from build123d import *

# Parameters (mm, degrees)
SKETCH1_R           = 7
BOSS_EXTRUDE1_DEPTH = 1
SKETCH2_R           = 6.475
BOSS_EXTRUDE2_DEPTH = 2
SKETCH3_R           = 4.75
CUT_EXTRUDE1_DEPTH  = 11.344080433
CHAMFER1_SIZE       = 0.5


with BuildPart() as part:
    # Sketch1 → Boss-Extrude1 (new body)
    with BuildSketch(Plane(origin=(0, 0, 0), x_dir=(1, 0, 0), z_dir=(0, 1, 0))):
        with Locations(Location((0, 0, 0), (0, 0, 270))):
            Circle(SKETCH1_R)
    extrude(amount=BOSS_EXTRUDE1_DEPTH)

    # Sketch2 → Boss-Extrude2 (add)
    with BuildSketch(Plane(origin=(0, 1, 0), x_dir=(1, 0, 0), z_dir=(0, 1, 0))):
        with Locations(Location((0, 0, 0), (0, 0, 270))):
            Circle(SKETCH2_R)
    extrude(amount=BOSS_EXTRUDE2_DEPTH)

    # Sketch3 → Cut-Extrude1 (cut, through all)
    with BuildSketch(Plane.XZ):
        with Locations(Location((0, 0, 0), (0, 0, 270))):
            Circle(SKETCH3_R)
    extrude(amount=-CUT_EXTRUDE1_DEPTH, mode=Mode.SUBTRACT)

    # Chamfer1
    chamfer1_edges = [part.edges().sort_by_distance(p)[0] for p in [
        (0, 0, 4.75),
    ]]
    chamfer(chamfer1_edges, length=CHAMFER1_SIZE)


solid = part.part
Source: CAD feature listing. Evaluate the final solid. Frame: model axes, mm. A direction names the side the tool comes from. Coordinates: 2 decimals unless noted, no trailing zeros. Loops run counter-clockwise (first coordinate to the right, second up) from the corner with the lowest first, then second, coordinate; pieces in that order, holes last. Notation, with made-up numbers: M -37.75,-15 L 5.25,-15 A8 ccw 5.25,-8 Z; hole C 0.5,83 d7. An arc over 180 degrees is marked long. Answer in a Markdown table with one row per item.
Q1. Section D-D on y = 2.45. Return the cut outline in (x, z) (3 decimals).
Answers below:
| item | result |
|---|---|
| outline | C 0,0 d12.95; hole C 0,0 d9.5 |
Q2. Section B-B on x = 0. Return the cut outline in (y, z) (3 decimals).
Answers below:
| item | result |
|---|---|
| outline | M 0,-7 L 1,-7 L 1,-6.475 L 3,-6.475 L 3,-4.75 L 0.5,-4.75 L 0,-5.25 Z; M 0,5.25 L 0.5,4.75 L 3,4.75 L 3,6.475 L 1,6.475 L 1,7 L 0,7 Z |
Q3. Section C-C on x = 6. Return the cut outline in (y, z), plus the area to 3 significant figures.
Answers below:
| item | result |
|---|---|
| outline | M 0,-3.61 L 1,-3.61 L 1,-2.43 L 3,-2.43 L 3,2.43 L 1,2.43 L 1,3.61 L 0,3.61 Z |
| area | 16.9 mm^2 |
Q4. Section A-A on z = 0. Return the cut outline in (x, y) (3 decimals), plus the area to 4 significant figures.
Answers below:
| item | result |
|---|---|
| outline | M -7,0 L -5.25,0 L -4.75,0.5 L -4.75,3 L -6.475,3 L -6.475,1 L -7,1 Z; M 4.75,0.5 L 5.25,0 L 7,0 L 7,1 L 6.475,1 L 6.475,3 L 4.75,3 Z |
| area | 11.15 mm^2 |
Q5. Ray query, probe 1 along X at (y, z) = (2, 0) (3 decimals); probe 2 along X at (y, z) = (1.65, -1.25); probe 3 along Z at (x, y) = (4, 2.2). Return the intervals inside material, ascending. Write a range as from..to.
Answers below:
| item | result |
|---|---|
| probe 1 | x = -6.475..-4.75, 4.75..6.475 |
| probe 2 | x = -6.35..-4.58, 4.58..6.35 |
| probe 3 | z = -5.09..-2.56, 2.56..5.09 |
Q6. Set-up query: faces 4 (the flat face through (5, 0, 3)), 5 (the flat face through (3, 1, 6)). Return all of +Z, -Z, +X, -X, +Y, -Y with unobstructed straight access to the full face (end or side cutting, diameter ignored); none if empty.
Answers below:
| item | result |
|---|---|
| face 4 | +Z, -Z, +X, -X, -Y |
| face 5 | +Y |
Q7. First-contact query: pin 1 (1.5 mm diameter, centred on x = -2.5, y = 2.5, fed in from -Z); pin 2 (1.5 mm diameter, centred on x = -2, y = 1.5, fed in from +Z). Flat tips, straight axial feed; report the tip coordinate or a pass-through.
Answers below:
| item | result |
|---|---|
| pin 1 | stops at z = -6.23 |
| pin 2 | stops at z = 6.85 |
Q8. Draft query along X for faces 1 (the cylindrical face through (-6.834, 0.493, -1.517)), 2 (the cylindrical face through (-2.89, 1.73, 3.77)), 3 (the flat face through (5, 3, -1)). Return one class per face: pulls with the +X half, pulls with the -X half, needs draft (parallel to the pull), parting line crosses it, or undercut.
Answers below:
| item | result |
|---|---|
| face 1 | parting line crosses it |
| face 2 | undercut |
| face 3 | needs draft |
